from build123d import *

# Parameters (mm, degrees)
F0_W     = 76.2
F0_H     = 12.7
F1_DEPTH = 127
F2_W     = 6.35
F2_H     = 6.35
F3_DEPTH = 76.2
F5_DEPTH = 127.001


with BuildPart() as f1:
    # F0 (on Top) → F1 (new body)
    with BuildSketch(Plane.XY):
        with Locations((0, -19.05)):
            Rectangle(F0_W, F0_H)
    extrude(amount=F1_DEPTH)

    # F2 (on face) → F3 (cut, through all)
    with BuildSketch(Plane.YZ.offset(38.1)):
        with Locations((-15.875, 9.525)):
            Rectangle(F2_W, F2_H)
    extrude(amount=-F3_DEPTH, mode=Mode.SUBTRACT)

    # F4 (on face) → F5 (cut, through all)
    with BuildSketch(Plane.XY.offset(127)):
        Polygon((-38.1, -12.7), (-38.1, -25.4), (-25.4, -12.7), align=None)
        Polygon((25.4, -12.7), (38.1, -25.4), (38.1, -12.7), align=None)
    extrude(amount=-F5_DEPTH, mode=Mode.SUBTRACT)


solid = f1.part
Could you check a few things on this model? Use its own coordinates, in mm. A direction names the side the tool comes from. Coordinates: 2 decimals unless noted, no trailing zeros. Order: outer loops, then holes, each group sorted by start corner. A loop starts at its lowest first (then second) coordinate and runs counter-clockwise, first axis right, second up. Notation, with made-up numbers: (50, 56.5) -> (97, 56.5) arc R13 cw to (97, 80.5) -> close; hole circle Ø11 at (55, 63). An arc over 180 degrees is marked (long way). One line per question, with ' | ' between items.
Q1. Thinking about a two-plate mould opening in Z: for faces 3 (the face through (0, -16, 12.7)), 4 (the face through (0, -19.05, 9)), 5 (the face through (31.7, -19, 64.4)), 6 (the face through (-1, -19, 127)), which applies, pulls with the +Z half, pulls with the -Z half, needs draft (parallel to the pull), parting line crosses it, or undercut?
Return value:
face 3: undercut | face 4: undercut | face 5: needs draft | face 6: pulls with the +Z half
Q2. I'm going to push flat-ended pins straight in: P1, Ø5, axis at x = -13, z = 9.5, coming from the +Y side; P2, Ø2, axis at x = -28, y = -18.5, coming from the -Z side; P3, Ø2, axis at y = -14, z = 93.5, coming from the +X side; P4, Ø5, axis at y = -19.5, z = 60, coming from the -X side. Where does each tip first touch, or does it pass through?
Return value:
P1: y = -19.05 | P2: z = 0 | P3: x = 27.7 | P4: x = -34.7
Q3. On a 3-axis mill with a long thin cutter (end or side, diameter ignored), from which of +Z, -Z, +X, -X, +Y, -Y can I reach the whole of each face in a straight line? I mean faces 1 (the face through (0, -16, 6.35)), 2 (the face through (-31.8, -19.1, 64.4)). Say none if no direction works.
Return value:
face 1: +X, -X, +Y | face 2: +Z, -Z, -X, +Y
Q4. Imagine slicing it at A-A on y = -16. Please give me the cut outline in (x, z), and give its area (3 significant figures).
Return value:
outline: (-28.7, 0) -> (28.7, 0) -> (28.7, 6.35) -> (-28.7, 6.35) -> close; (-28.7, 12.7) -> (28.7, 12.7) -> (28.7, 127) -> (-28.7, 127) -> close | area: 6,930 mm²
Q5. Imagine slicing it at B-B on x = -4.5. Please give me the cut outline in (y, z), and give its area (3 significant figures).
Return value:
outline: (-25.4, 0) -> (-12.7, 0) -> (-12.7, 6.35) -> (-19.05, 6.35) -> (-19.05, 12.7) -> (-12.7, 12.7) -> (-12.7, 127) -> (-25.4, 127) -> close | area: 1,570 mm²
Q6. Imagine slicing it at D-D on y = -23.25. Please give me the cut outline in (x, z).
Return value:
outline: (-35.95, 0) -> (35.95, 0) -> (35.95, 127) -> (-35.95, 127) -> close
Q7. Imagine slicing it at C-C on z = 40.5. Please give me the cut outline in (x, y), and give its area (3 significant figures).
Return value:
outline: (-38.1, -25.4) -> (38.1, -25.4) -> (25.4, -12.7) -> (-25.4, -12.7) -> close | area: 806 mm²
Q8. If I drill on L1, parallel to Z at x = 5, y = -15.25; L2, parallel to Y at x = -8, z = 12, over which ranges is the centre line in solid material (lowest first)?
Return value:
L1: 0 to 6.35, 12.7 to 127 | L2: -25.4 to -19.05
